Here's how the part is built. I have some questions about the finished solid (model axes, mm). Face numbers are marked on the shaded views. A direction names the side the tool comes from. Give positions to 0.01 mm unless a question says otherwise; leave off trailing zeros. Loops run counter-clockwise (first coordinate to the right, second up) from the corner with the lowest first, then second, coordinate; pieces in that order, holes last.
Q1. If we section it at B-B (x = 4.95): Please give me the cut outline in (y, z), plus the area to 3 significant figures.
Q2. For the marked faces 1, 2, 3 and 4, which set-ups out of +Z, -Z, +X, -X, +Y, -Y let a thin tool reach every point of the face, with its end or its side?
Q3. Will these pins go through, and if not, where does the flat tip stop? P1, Ø1.7, axis at x = -2.5, z = 14.5, coming from the +Y side; P2, Ø5.5, axis at x = -2, y = -23.5, coming from the -Z side; P3, Ø8, axis at x = -5.5, z = -9.5, coming from the -Y side.
Q4. I need wall thicknesses on line 1 (Y direction, x = 4.95, z = 11.3); line 2 (X direction, y = 24.3, z = 10.9); line 3 (Y direction, x = -1, z = -5.5). Which ranges of each line are inside material? Lowest first, please.
Q5. If we section it at C-C (x = -1.5): Please give me the cut outline in (y, z), plus the area to 3 significant figures.
Q6. If we section it at D-D (z = -11.5): Please give me the cut outline in (x, y).
Q7. If we section it at A-A (y = 24.3): Please give me the cut outline in (x, z).
from build123d import *

# Parameters (mm, degrees)
SKETCH4_W               = 19.9
SKETCH4_H               = 40.4
BOSS_EXTRUDE3_DEPTH     = 17.85
SKETCH6_W               = 19.9
SKETCH6_H               = 54
BOSS_EXTRUDE4_DEPTH     = 3
CUT_EXTRUDE2_DEPTH      = 34.861851692
CUT_EXTRUDE2_DEPTH_BACK = 34.861851692
SKETCH1_R               = 2.5


with BuildPart() as part:
    # Sketch4 → Boss-Extrude3 (new, symmetric)
    with BuildSketch(Plane.XY):
        Rectangle(SKETCH4_W, SKETCH4_H)
    extrude(amount=BOSS_EXTRUDE3_DEPTH, both=True)

    # Sketch6 → Boss-Extrude4 (add)
    with BuildSketch(Plane(origin=(0, 0, 9.05), x_dir=(-1, 0, 0), z_dir=(0, 0, -1))):
        Rectangle(SKETCH6_W, SKETCH6_H)
    extrude(amount=-BOSS_EXTRUDE4_DEPTH)

    # Sketch1 → Cut-Extrude2 (cut, two sides: drawn at the far end of the back side and taken through both)
    with BuildSketch(Plane.XY.offset(-CUT_EXTRUDE2_DEPTH_BACK)):
        with Locations((4.95, -24.3)):
            Circle(SKETCH1_R)
        with Locations((-4.95, -24.3)):
            Circle(SKETCH1_R)
        with Locations((-4.95, 24.3)):
            Circle(SKETCH1_R)
        with Locations((4.95, 24.3)):
            Circle(SKETCH1_R)
    extrude(amount=CUT_EXTRUDE2_DEPTH + CUT_EXTRUDE2_DEPTH_BACK, mode=Mode.SUBTRACT)


solid = part.part
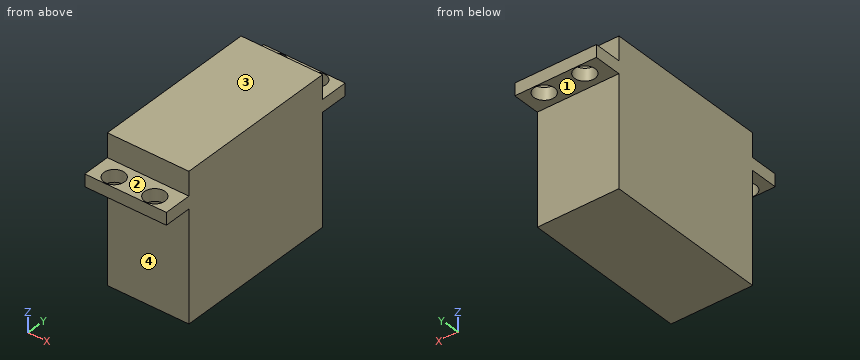
Check sheet entries:
1. outline: (-27, 9.05) - (-26.8, 9.05) - (-26.8, 12.05) - (-27, 12.05) - close; (-21.8, 9.05) - (-20.2, 9.05) - (-20.2, -17.85) - (20.2, -17.85) - (20.2, 9.05) - (21.8, 9.05) - (21.8, 12.05) - (20.2, 12.05) - (20.2, 17.85) - (-20.2, 17.85) - (-20.2, 12.05) - (-21.8, 12.05) - close; (26.8, 9.05) - (27, 9.05) - (27, 12.05) - (26.8, 12.05) - close
1. area: 1,450 mm2
2. face 1: -Z, +X, -X, +Y
2. face 2: +Z, +X, -X, -Y
2. face 3: +Z, +X, -X, +Y, -Y
2. face 4: -Z, +X, -X, -Y
3. P1: stops at y = 20.2
3. P2: stops at z = 9.05
3. P3: stops at y = -20.2
4. line 1: y = -27 to -26.8, -21.8 to 21.8, 26.8 to 27
4. line 2: x = -9.95 to -7.45, -2.45 to 2.45, 7.45 to 9.95
4. line 3: y = -20.2 to 20.2
5. outline: (-27, 9.05) - (-20.2, 9.05) - (-20.2, -17.85) - (20.2, -17.85) - (20.2, 9.05) - (27, 9.05) - (27, 12.05) - (20.2, 12.05) - (20.2, 17.85) - (-20.2, 17.85) - (-20.2, 12.05) - (-27, 12.05) - close
5. area: 1,480 mm2
6. outline: (-9.95, -20.2) - (9.95, -20.2) - (9.95, 20.2) - (-9.95, 20.2) - close
7. outline: (-9.95, 9.05) - (-7.45, 9.05) - (-7.45, 12.05) - (-9.95, 12.05) - close; (-2.45, 9.05) - (2.45, 9.05) - (2.45, 12.05) - (-2.45, 12.05) - close; (7.45, 9.05) - (9.95, 9.05) - (9.95, 12.05) - (7.45, 12.05) - close
